Job drawing, mm, ordinate dimensions from the low corner. One solid piece. Give positions to 0.01 mm unless a question says otherwise; leave off trailing zeros. Write each loop counter-clockwise with the first axis right and the second up, starting at its lowest first coordinate (ties: lowest second). Pieces come first, ordered by that corner, then holes. Notation, with made-up numbers: M 10.5,88 L 48.5,88 A18 cw 48.5,97 Z; hole C 47.25,-21 d10. An arc over 180 degrees is marked long. Use CSV: the item, a comma, the result in double quotes. Start each with the question number.
Item 1: Cut at C-C (x = 12). List the corners of the cut face in (y, z).
Item 2: Drill centre lines: line 1 (X direction, y = 8.75, z = 5) (1 decimal); line 2 (X direction, y = 9.25, z = 0.75) (1 decimal); line 3 (Y direction, x = 8, z = 3.25) (1 decimal). Where is each one in solid material? Low to high. Write a range as [from, to].
Item 3: Mould opens along X. For the marked faces 1, 2 and 3 say: released by +X, released by -X, zero draft, split by the parting line, or undercut.
Item 4: Cut at A-A (z = 3.5). List the corners of the cut face in (x, y) (1 decimal).
Item 5: Pin check, flat tip, straight feed: pin 1 (3 mm diameter, centred on x = 11, z = 2.5, fed in from -Y) (1 decimal). Stop position of the tip, or through.
Item 6: Cut at B-B (y = 13). List the corners of the cut face in (x, z), then the cut area to 3 significant figures.
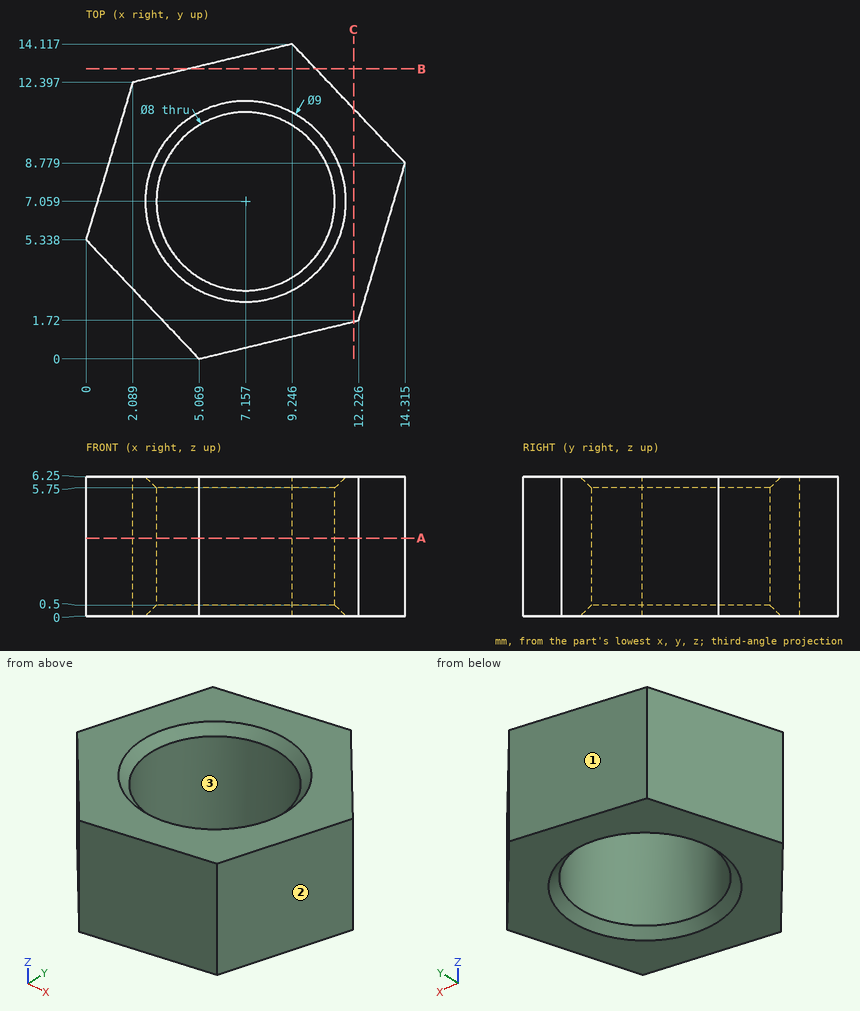
Worked answers:
1,outline,"M 1.67,0 L 11.22,0 L 11.22,6.25 L 1.67,6.25 Z"
2,line 1,"x = [1, 3.5], [10.8, 14.3]"
2,line 2,"x = [1.2, 3.8], [10.5, 13.9]"
2,line 3,"y = [0.7, 3.1], [11, 13.8]"
3,face 1,"released by -X"
3,face 2,"released by +X"
3,face 3,"undercut"
4,outline,"M 0,5.3 L 5.1,0 L 12.2,1.7 L 14.3,8.8 L 9.2,14.1 L 2.1,12.4 Z; hole C 7.2,7.1 d8"
5,pin 1,"stops at y = 1.1"
6,outline,"M 4.6,0 L 10.31,0 L 10.31,6.25 L 4.6,6.25 Z"
6,area,"35.7 mm^2"
